from build123d import *

# Parameters (mm, degrees)
SKETCH9_W           = 40
SKETCH9_H           = 30
BOSS_EXTRUDE2_DEPTH = 30
SKETCH10_R          = 10
CUT_EXTRUDE1_DEPTH  = 15
SKETCH11_R          = 8
SKETCH11_R_2        = 4
CUT_EXTRUDE2_DEPTH  = 5
CUT_EXTRUDE3_DEPTH  = 101
SKETCH12_R          = 3
CUT_EXTRUDE4_DEPTH  = 101


with BuildPart() as part:
    # Sketch9 → Boss-Extrude2 (new body)
    with BuildSketch(Plane.XY):
        with Locations((20, -15)):
            Rectangle(SKETCH9_W, SKETCH9_H)
    extrude(amount=BOSS_EXTRUDE2_DEPTH)

    # Sketch10 → Cut-Extrude1 (cut)
    with BuildSketch(Plane(origin=(40, 0, 0), x_dir=(0, 0, -1), z_dir=(1, 0, 0))):
        with Locations(Location((-15, -15, 0), (0, 0, 90))):
            Circle(SKETCH10_R)
    extrude(amount=-CUT_EXTRUDE1_DEPTH, mode=Mode.SUBTRACT)

    # Sketch11 → Cut-Extrude2 (cut)
    with BuildSketch(Plane.XY.offset(30)):
        with Locations((12.5, -15)):
            Circle(SKETCH11_R)
        with Locations((12.5, -15)):
            Circle(SKETCH11_R_2, mode=Mode.SUBTRACT)
    cut_extrude2 = extrude(amount=-CUT_EXTRUDE2_DEPTH, mode=Mode.SUBTRACT)

    # Sketch11_3 → Cut-Extrude3 (cut)
    with BuildSketch(Plane.XY.offset(30)):
        with BuildLine():
            ThreePointArc((16.5, -15), (14.196621585, -11.377642315), (9.939262401, -11.927114882))
            Line((9.939262401, -11.927114882), (15.060737599, -18.072885118))
            ThreePointArc((15.060737599, -18.072885118), (16.122357685, -16.696621585), (16.5, -15))
        make_face()
        with BuildLine():
            Line((15.060737599, -18.072885118), (9.939262401, -11.927114882))
            ThreePointArc((9.939262401, -11.927114882), (9.427114882, -17.560737599), (15.060737599, -18.072885118))
        make_face()
    extrude(amount=-CUT_EXTRUDE3_DEPTH, mode=Mode.SUBTRACT)

    # Sketch12 → Cut-Extrude4 (cut)
    with BuildSketch(Plane.XY.offset(30)):
        with Locations((32.1, -15)):
            Circle(SKETCH12_R)
    extrude(amount=-CUT_EXTRUDE4_DEPTH, mode=Mode.SUBTRACT)

    # Mirror1: Cut-Extrude2 across plane
    add(cut_extrude2.mirror(Plane(origin=(0, 0, 15), x_dir=(1, 0, 0), z_dir=(0, 0, -1))), mode=Mode.SUBTRACT)


solid = part.part
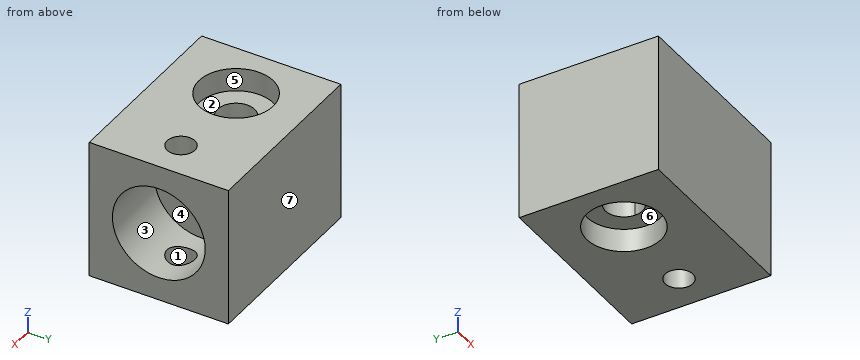
Design review of the part built by this model. Coordinates are the model's own, in mm. Face numbers are marked on the shaded views. A direction names the side the tool comes from. Coordinates: 2 decimals unless noted, no trailing zeros. Loops run counter-clockwise (first coordinate to the right, second up) from the corner with the lowest first, then second, coordinate; pieces in that order, holes last.
Item 1: Wall thickness on L1, parallel to Y at x = 32.1, z = 27.85; L2, parallel to Z at x = 28, y = -14.5; L3, parallel to Z at x = 6, y = -10.5: over which ranges is each line inside the solid? List them lowest first.
Completed:
L1: y = -30 to -18, -12 to 0
L2: z = 0 to 5.01, 24.99 to 30
L3: z = 5 to 25
Item 2: Clearance check with flat-ended pins moving along their axes: pin 1 (1 mm diameter, centred on y = -16, z = 20, fed in from -X); pin 2 (6 mm diameter, centred on y = -10.5, z = 18, fed in from +X); pin 3 (5 mm diameter, centred on x = 16, y = -18, fed in from +Z). State where each tip first meets the part, or that it passes through.
Completed:
pin 1: stops at x = 0
pin 2: stops at x = 25
pin 3: stops at z = 25
Item 3: Add section A-A (x = 12.5). Write out the cut boundary in (y, z).
Completed:
outline: (-30, 0) - (-23, 0) - (-23, 5) - (-19, 5) - (-19, 25) - (-23, 25) - (-23, 30) - (-30, 30) - close; (-11, 5) - (-7, 5) - (-7, 0) - (0, 0) - (0, 30) - (-7, 30) - (-7, 25) - (-11, 25) - close
Item 4: Draft analysis for pull direction Z (two halves, no side actions). For the marked faces 1, 2 and 3, state which applies: pulls with the +Z half, pulls with the -Z half, needs draft (parallel to the pull), parting line crosses it, or undercut.
Completed:
face 1: needs draft
face 2: pulls with the +Z half
face 3: undercut
Item 5: Add section C-C (x = 25.5). Write out the cut boundary in (y, z), and give its area (3 significant figures).
Completed:
outline: (-30, 0) - (0, 0) - (0, 30) - (-30, 30) - close; hole circle Ø20 at (-15, 15)
area: 586 mm2
Item 6: For the marked faces 4, 5, 6 and 7, list the 3-axis set-ups (+Z, -Z, +X, -X, +Y, -Y) from which the entire face can be reached by the end or side of a thin tool; tool diameter is ignored.
Completed:
face 4: +X
face 5: +Z
face 6: -Z
face 7: +Z, -Z, +X, -X, +Y
Item 7: Add section D-D (z = 9). Write out the cut boundary in (x, y), and give its area (3 significant figures).
Completed:
outline: (0, -30) - (40, -30) - (40, -23) - (25, -23) - (25, -7) - (40, -7) - (40, 0) - (0, 0) - close; hole circle Ø8 at (12.5, -15)
area: 910 mm2
Item 8: Add section B-B (z = 15). Write out the cut boundary in (x, y).
Completed:
outline: (0, -30) - (40, -30) - (40, -25) - (25, -25) - (25, -5) - (40, -5) - (40, 0) - (0, 0) - close; hole circle Ø8 at (12.5, -15)
